```python
from build123d import *

# Parameters (mm, degrees)
SKETCH_1_R          = 19
EXTRUDE_1_DEPTH     = 3
CUT_EXTRUDE_1_REACH = 5
SKETCH_2_R          = 2.1
CUT_EXTRUDE_2_REACH = 5
SKETCH_3_R          = 10


with BuildPart() as part:
    # ｽｹｯﾁ1 → ﾎﾞｽ - 押し出し1 (new body)
    with BuildSketch(Plane(origin=(0, 0, 0), x_dir=(1, 0, 0), z_dir=(0, 1, 0))):
        Circle(SKETCH_1_R)
    extrude(amount=EXTRUDE_1_DEPTH)

    # ｽｹｯﾁ2 → ｶｯﾄ - 押し出し1 (cut, up to next)
    with BuildSketch(Plane(origin=(0, 3, 0), x_dir=(1, 0, 0), z_dir=(0, 1, 0)), mode=Mode.PRIVATE) as cut_extrude_1_sk1:
        with Locations((0, 15)):
            Circle(SKETCH_2_R)
    cut_extrude_1_tool1 = extrude(cut_extrude_1_sk1.sketch, amount=-CUT_EXTRUDE_1_REACH, mode=Mode.PRIVATE) & part.part
    add(cut_extrude_1_tool1.solids().sort_by_distance((0, 3, -15))[0], mode=Mode.SUBTRACT)
    # ｽｹｯﾁ2 → ｶｯﾄ - 押し出し1 (cut, up to next)
    with BuildSketch(Plane(origin=(0, 3, 0), x_dir=(1, 0, 0), z_dir=(0, 1, 0)), mode=Mode.PRIVATE) as cut_extrude_1_sk2:
        with Locations((7.5, 12.990381057)):
            Circle(SKETCH_2_R)
    cut_extrude_1_tool2 = extrude(cut_extrude_1_sk2.sketch, amount=-CUT_EXTRUDE_1_REACH, mode=Mode.PRIVATE) & part.part
    add(cut_extrude_1_tool2.solids().sort_by_distance((7.5, 3, -12.990381))[0], mode=Mode.SUBTRACT)
    # ｽｹｯﾁ2 → ｶｯﾄ - 押し出し1 (cut, up to next)
    with BuildSketch(Plane(origin=(0, 3, 0), x_dir=(1, 0, 0), z_dir=(0, 1, 0)), mode=Mode.PRIVATE) as cut_extrude_1_sk3:
        with Locations((12.990381057, 7.5)):
            Circle(SKETCH_2_R)
    cut_extrude_1_tool3 = extrude(cut_extrude_1_sk3.sketch, amount=-CUT_EXTRUDE_1_REACH, mode=Mode.PRIVATE) & part.part
    add(cut_extrude_1_tool3.solids().sort_by_distance((12.990381, 3, -7.5))[0], mode=Mode.SUBTRACT)
    # ｽｹｯﾁ2 → ｶｯﾄ - 押し出し1 (cut, up to next)
    with BuildSketch(Plane(origin=(0, 3, 0), x_dir=(1, 0, 0), z_dir=(0, 1, 0)), mode=Mode.PRIVATE) as cut_extrude_1_sk4:
        with Locations((15, 0)):
            Circle(SKETCH_2_R)
    cut_extrude_1_tool4 = extrude(cut_extrude_1_sk4.sketch, amount=-CUT_EXTRUDE_1_REACH, mode=Mode.PRIVATE) & part.part
    add(cut_extrude_1_tool4.solids().sort_by_distance((15, 3, 0))[0], mode=Mode.SUBTRACT)
    # ｽｹｯﾁ2 → ｶｯﾄ - 押し出し1 (cut, up to next)
    with BuildSketch(Plane(origin=(0, 3, 0), x_dir=(1, 0, 0), z_dir=(0, 1, 0)), mode=Mode.PRIVATE) as cut_extrude_1_sk5:
        with Locations((12.990381057, -7.5)):
            Circle(SKETCH_2_R)
    cut_extrude_1_tool5 = extrude(cut_extrude_1_sk5.sketch, amount=-CUT_EXTRUDE_1_REACH, mode=Mode.PRIVATE) & part.part
    add(cut_extrude_1_tool5.solids().sort_by_distance((12.990381, 3, 7.5))[0], mode=Mode.SUBTRACT)
    # ｽｹｯﾁ2 → ｶｯﾄ - 押し出し1 (cut, up to next)
    with BuildSketch(Plane(origin=(0, 3, 0), x_dir=(1, 0, 0), z_dir=(0, 1, 0)), mode=Mode.PRIVATE) as cut_extrude_1_sk6:
        with Locations((7.5, -12.990381057)):
            Circle(SKETCH_2_R)
    cut_extrude_1_tool6 = extrude(cut_extrude_1_sk6.sketch, amount=-CUT_EXTRUDE_1_REACH, mode=Mode.PRIVATE) & part.part
    add(cut_extrude_1_tool6.solids().sort_by_distance((7.5, 3, 12.990381))[0], mode=Mode.SUBTRACT)
    # ｽｹｯﾁ2 → ｶｯﾄ - 押し出し1 (cut, up to next)
    with BuildSketch(Plane(origin=(0, 3, 0), x_dir=(1, 0, 0), z_dir=(0, 1, 0)), mode=Mode.PRIVATE) as cut_extrude_1_sk7:
        with Locations((0, -15)):
            Circle(SKETCH_2_R)
    cut_extrude_1_tool7 = extrude(cut_extrude_1_sk7.sketch, amount=-CUT_EXTRUDE_1_REACH, mode=Mode.PRIVATE) & part.part
    add(cut_extrude_1_tool7.solids().sort_by_distance((0, 3, 15))[0], mode=Mode.SUBTRACT)
    # ｽｹｯﾁ2 → ｶｯﾄ - 押し出し1 (cut, up to next)
    with BuildSketch(Plane(origin=(0, 3, 0), x_dir=(1, 0, 0), z_dir=(0, 1, 0)), mode=Mode.PRIVATE) as cut_extrude_1_sk8:
        with Locations((-7.5, -12.990381057)):
            Circle(SKETCH_2_R)
    cut_extrude_1_tool8 = extrude(cut_extrude_1_sk8.sketch, amount=-CUT_EXTRUDE_1_REACH, mode=Mode.PRIVATE) & part.part
    add(cut_extrude_1_tool8.solids().sort_by_distance((-7.5, 3, 12.990381))[0], mode=Mode.SUBTRACT)
    # ｽｹｯﾁ2 → ｶｯﾄ - 押し出し1 (cut, up to next)
    with BuildSketch(Plane(origin=(0, 3, 0), x_dir=(1, 0, 0), z_dir=(0, 1, 0)), mode=Mode.PRIVATE) as cut_extrude_1_sk9:
        with Locations((-12.990381057, -7.5)):
            Circle(SKETCH_2_R)
    cut_extrude_1_tool9 = extrude(cut_extrude_1_sk9.sketch, amount=-CUT_EXTRUDE_1_REACH, mode=Mode.PRIVATE) & part.part
    add(cut_extrude_1_tool9.solids().sort_by_distance((-12.990381, 3, 7.5))[0], mode=Mode.SUBTRACT)
    # ｽｹｯﾁ2 → ｶｯﾄ - 押し出し1 (cut, up to next)
    with BuildSketch(Plane(origin=(0, 3, 0), x_dir=(1, 0, 0), z_dir=(0, 1, 0)), mode=Mode.PRIVATE) as cut_extrude_1_sk10:
        with Locations((-15, 0)):
            Circle(SKETCH_2_R)
    cut_extrude_1_tool10 = extrude(cut_extrude_1_sk10.sketch, amount=-CUT_EXTRUDE_1_REACH, mode=Mode.PRIVATE) & part.part
    add(cut_extrude_1_tool10.solids().sort_by_distance((-15, 3, 0))[0], mode=Mode.SUBTRACT)
    # ｽｹｯﾁ2 → ｶｯﾄ - 押し出し1 (cut, up to next)
    with BuildSketch(Plane(origin=(0, 3, 0), x_dir=(1, 0, 0), z_dir=(0, 1, 0)), mode=Mode.PRIVATE) as cut_extrude_1_sk11:
        with Locations((-12.990381057, 7.5)):
            Circle(SKETCH_2_R)
    cut_extrude_1_tool11 = extrude(cut_extrude_1_sk11.sketch, amount=-CUT_EXTRUDE_1_REACH, mode=Mode.PRIVATE) & part.part
    add(cut_extrude_1_tool11.solids().sort_by_distance((-12.990381, 3, -7.5))[0], mode=Mode.SUBTRACT)
    # ｽｹｯﾁ2 → ｶｯﾄ - 押し出し1 (cut, up to next)
    with BuildSketch(Plane(origin=(0, 3, 0), x_dir=(1, 0, 0), z_dir=(0, 1, 0)), mode=Mode.PRIVATE) as cut_extrude_1_sk12:
        with Locations((-7.5, 12.990381057)):
            Circle(SKETCH_2_R)
    cut_extrude_1_tool12 = extrude(cut_extrude_1_sk12.sketch, amount=-CUT_EXTRUDE_1_REACH, mode=Mode.PRIVATE) & part.part
    add(cut_extrude_1_tool12.solids().sort_by_distance((-7.5, 3, -12.990381))[0], mode=Mode.SUBTRACT)

    # ｽｹｯﾁ3 → ｶｯﾄ - 押し出し2 (cut, up to next)
    with BuildSketch(Plane(origin=(0, 3, 0), x_dir=(1, 0, 0), z_dir=(0, 1, 0)), mode=Mode.PRIVATE) as cut_extrude_2_sk1:
        Circle(SKETCH_3_R)
    cut_extrude_2_tool1 = extrude(cut_extrude_2_sk1.sketch, amount=-CUT_EXTRUDE_2_REACH, mode=Mode.PRIVATE) & part.part
    add(cut_extrude_2_tool1.solids().sort_by_distance((0, 3, 0))[0], mode=Mode.SUBTRACT)


solid = part.part
```
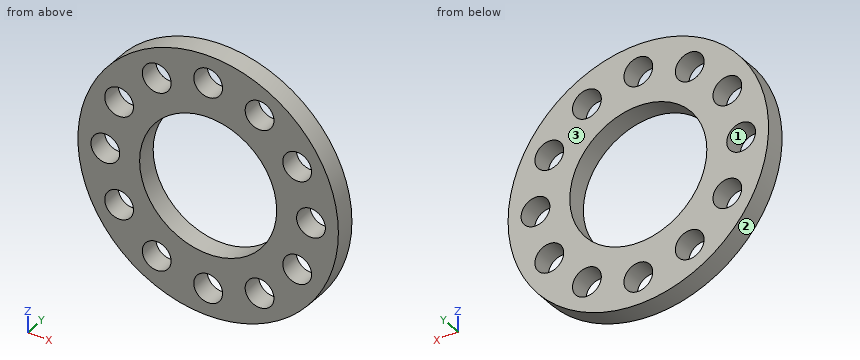
Here's how the part is built. I have some questions about the finished solid (model axes, mm). Face numbers are marked on the shaded views. Coordinates: 2 decimals unless noted, no trailing zeros. Write each loop counter-clockwise with the first axis right and the second up, starting at its lowest first coordinate (ties: lowest second). Pieces come first, ordered by that corner, then holes. Notation, with made-up numbers: (75, 22) -> (82, 22) arc R20 cw to (82, 37) -> close; hole circle Ø7 at (84.5, 73.5). An arc over 180 degrees is marked (long way). Use a Markdown table: item, result. Add a question column.
(1) If we section it at A-A, the plane z = 0: Write out the boundary of the cut face in (x, y).
(2) If we section it at B-B, the plane x = 7.5: Write out the boundary of the cut face in (y, z), and give its area (3 significant figures).
(3) If we section it at D-D, the plane y = 1.9: State how many separate pieces and enclosed holes the cut face has, and give its area (3 significant figures).
(4) We'd pull the mould along X, two halves only. Please class the marked faces 1, 2 and 3: +X half, -X half, draft (parallel to the pull), parting line (faces both ways), or undercut.
(5) I'm going to push flat-ended pins straight in: P1, Ø1, axis at y = 2, z = -6, coming from the -X side; P2, Ø5.5, axis at x = 0, z = 15, coming from the -Y side. Where does each tip first touch, or does it pass through?
(6) If we section it at C-C, the plane z = 16: Write out the boundary of the cut face in (x, y), and give its area (3 significant figures).
(7) Please list where these lines run through material, in increasing order: line 1 (Z direction, x = 11.5, y = 2.1); line 2 (X direction, y = 1.4, z = -6.5); line 3 (X direction, y = 1.65, z = 7.5).
Outcome:
| question | item | result |
|---|---|---|
| 1 | outline | (-19, 0) -> (-17.1, 0) -> (-17.1, 3) -> (-19, 3) -> close; (-12.9, 0) -> (-10, 0) -> (-10, 3) -> (-12.9, 3) -> close; (10, 0) -> (12.9, 0) -> (12.9, 3) -> (10, 3) -> close; (17.1, 0) -> (19, 0) -> (19, 3) -> (17.1, 3) -> close |
| 2 | outline | (0, -17.46) -> (3, -17.46) -> (3, -15.09) -> (0, -15.09) -> close; (0, -10.89) -> (3, -10.89) -> (3, -6.61) -> (0, -6.61) -> close; (0, 6.61) -> (3, 6.61) -> (3, 10.89) -> (0, 10.89) -> close; (0, 15.09) -> (3, 15.09) -> (3, 17.46) -> (0, 17.46) -> close |
| 2 | area | 39.9 mm^2 |
| 3 | separate pieces | 1 |
| 3 | enclosed holes | 13 |
| 3 | area | 654 mm^2 |
| 4 | face 1 | undercut |
| 4 | face 2 | parting line |
| 4 | face 3 | draft |
| 5 | P1 | stops at x = -18.19 |
| 5 | P2 | stops at y = 0 |
| 6 | outline | (-10.25, 0) -> (-1.85, 0) -> (-1.85, 3) -> (-10.25, 3) -> close; (1.85, 0) -> (10.25, 0) -> (10.25, 3) -> (1.85, 3) -> close |
| 6 | area | 50.4 mm^2 |
| 7 | line 1 | z = -15.12 to -8.98, -6.02 to 6.02, 8.98 to 15.12 |
| 7 | line 2 | x = -17.85 to -14.84, -11.14 to -7.6, 7.6 to 11.14, 14.84 to 17.85 |
| 7 | line 3 | x = -17.46 to -15.09, -10.89 to -6.61, 6.61 to 10.89, 15.09 to 17.46 |
